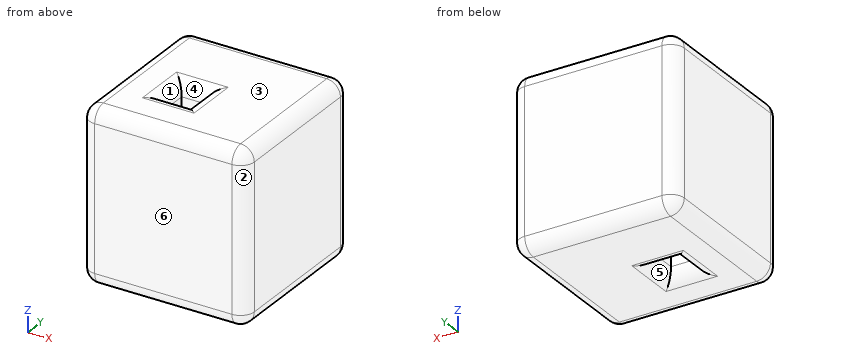
from build123d import *

# Parameters (mm, degrees)
F0_W     = 24
F0_H     = 24
F0_W_2   = 3.526274
F0_H_2   = 3.947003
F1_DEPTH = 25
F2_R     = 2
F3_R     = 2


with BuildPart() as f1:
    # F0 (on Top) → F1 (new body)
    with BuildSketch(Plane.XY):
        with Locations((-32.678599, -18.286714)):
            Rectangle(F0_W, F0_H)
        with Locations((-35.5378, -20.619581)):
            Rectangle(F0_W_2, F0_H_2, mode=Mode.SUBTRACT)
    extrude(amount=F1_DEPTH)

    # F2
    f2_edges = [f1.edges().sort_by_distance(p)[0] for p in [
        (-44.678599, -6.286714, 12.5),
        (-32.678599, -6.286714, 25),
        (-20.678599, -6.286714, 12.5),
        (-32.678599, -6.286714, 0),
        (-44.678599, -30.286714, 12.5),
        (-44.678599, -18.286714, 0),
        (-44.678599, -18.286714, 25),
        (-32.678599, -30.286714, 25),
        (-20.678599, -18.286714, 25),
        (-20.678599, -30.286714, 12.5),
        (-20.678599, -18.286714, 0),
        (-32.678599, -30.286714, 0),
    ]]
    fillet(f2_edges, radius=F2_R)

    # F3
    f3_edges = [f1.edges().sort_by_distance(p)[0] for p in [
        (-33.774663, -20.619581, 25),
        (-35.5378, -22.593083, 0),
        (-35.5378, -18.64608, 25),
        (-37.300937, -20.619581, 25),
        (-35.5378, -22.593083, 25),
        (-37.300937, -20.619581, 0),
        (-35.5378, -18.64608, 0),
        (-33.774663, -20.619581, 0),
    ]]
    fillet(f3_edges, radius=F3_R)


solid = f1.part
Work out the finished part from the listing and answer in its coordinate system (mm). Face numbers are marked on the shaded views. A direction names the side the tool comes from. Coordinates: 2 decimals unless noted, no trailing zeros. Order: outer loops, then holes, each group sorted by start corner. A loop starts at its lowest first (then second) coordinate and runs counter-clockwise, first axis right, second up. Notation, with made-up numbers: (70.5, -34) - (89.5, -34) arc R23 ccw to (89.5, -1) - close; hole circle Ø8 at (19.5, 55). An arc over 180 degrees is marked (long way). Put each result on its own line as item: value. Start each with the question number.
1) For a pull along Y with two mould halves and no side action, classify the marked faces 1, 2 and 3 as released by +Y, released by -Y, zero draft, split by the parting line, or undercut.
2) Find the intervals of material crossed by line 1 (X direction, y = -21.5, z = 15.5); line 2 (Y direction, x = -36, z = 15.5); line 3 (X direction, y = -18.5, z = 24.25), in increasing order. Write a range as from..to.
3) Find section A-A (z = 7). Give the vertices of the cut face in (x, y), plus the area to 3 significant figures.
4) Find section C-C (y = -21). Give the vertices of the cut face in (x, z), plus the area to 3 significant figures.
5) Find section B-B (x = -35.25). Give the vertices of the cut face in (y, z).
6) For the marked faces 4, 5 and 6, determine the directions among +Z, -Z, +X, -X, +Y, -Y from which every point of the face is accessible in a straight line to the end or side of a thin tool.
Results list:
1. face 1: undercut
1. face 2: released by -Y
1. face 3: zero draft
2. line 1: x = -44.68..-37.3, -33.77..-20.68
2. line 2: y = -30.29..-22.59, -18.65..-6.29
2. line 3: x = -44.24..-37.74, -33.34..-21.12
3. outline: (-44.68, -28.29) arc R2 ccw to (-42.68, -30.29) - (-22.68, -30.29) arc R2 ccw to (-20.68, -28.29) - (-20.68, -8.29) arc R2 ccw to (-22.68, -6.29) - (-42.68, -6.29) arc R2 ccw to (-44.68, -8.29) - close; hole (-37.3, -22.59) - (-33.77, -22.59) - (-33.77, -18.65) - (-37.3, -18.65) - close
3. area: 559 mm^2
4. outline: (-44.68, 2) arc R2 ccw to (-42.68, 0) - (-39.3, 0) arc R2 ccw to (-37.3, 2) - (-37.3, 23) arc R2 ccw to (-39.3, 25) - (-42.68, 25) arc R2 ccw to (-44.68, 23) - close; (-33.77, 2) arc R2 ccw to (-31.77, 0) - (-22.68, 0) arc R2 ccw to (-20.68, 2) - (-20.68, 23) arc R2 ccw to (-22.68, 25) - (-31.77, 25) arc R2 ccw to (-33.77, 23) - close
4. area: 505 mm^2
5. outline: (-30.29, 2) arc R2 ccw to (-28.29, 0) - (-24.59, 0) arc R2 ccw to (-22.59, 2) - (-22.59, 23) arc R2 ccw to (-24.59, 25) - (-28.29, 25) arc R2 ccw to (-30.29, 23) - close; (-18.65, 2) arc R2 ccw to (-16.65, 0) - (-8.29, 0) arc R2 ccw to (-6.29, 2) - (-6.29, 23) arc R2 ccw to (-8.29, 25) - (-16.65, 25) arc R2 ccw to (-18.65, 23) - close
6. face 4: +Z
6. face 5: -Z
6. face 6: +Z, -Z, +X, -X, -Y
